Verification items for the finished model (mm, model axes). A direction names the side the tool comes from. Give positions to 0.01 mm unless a question says otherwise; leave off trailing zeros. Loops run counter-clockwise (first coordinate to the right, second up) from the corner with the lowest first, then second, coordinate; pieces in that order, holes last. Notation, with made-up numbers: M 20,-18 L 74,-18 A19 ccw 74,-11 Z; hole C 48.5,18 d9. An arc over 180 degrees is marked long. Use a Markdown table: item, result.
from build123d import *

# Parameters (mm, degrees)
SKETCH1_W           = 50
SKETCH1_H           = 101.6
BOSS_EXTRUDE1_DEPTH = 4
SKETCH2_R           = 3
CUT_EXTRUDE1_DEPTH  = 10
SKETCH3_R           = 6
CUT_EXTRUDE2_DEPTH  = 2


with BuildPart() as part:
    # Sketch1 → Boss-Extrude1 (new body)
    with BuildSketch(Plane(origin=(0, 0, 0), x_dir=(1, 0, 0), z_dir=(0, 1, 0))):
        Rectangle(SKETCH1_W, SKETCH1_H)
    extrude(amount=BOSS_EXTRUDE1_DEPTH)

    # Sketch2 → Cut-Extrude1 (cut)
    with BuildSketch(Plane(origin=(0, 4, 0), x_dir=(1, 0, 0), z_dir=(0, 1, 0))):
        with Locations((0, 20)):
            Circle(SKETCH2_R)
        with Locations((0, -20)):
            Circle(SKETCH2_R)
    extrude(amount=-CUT_EXTRUDE1_DEPTH, mode=Mode.SUBTRACT)

    # Sketch3 → Cut-Extrude2 (cut)
    with BuildSketch(Plane(origin=(0, 4, 0), x_dir=(1, 0, 0), z_dir=(0, 1, 0))):
        with Locations((0, 20)):
            Circle(SKETCH3_R)
        with Locations((0, -20)):
            Circle(SKETCH3_R)
    extrude(amount=-CUT_EXTRUDE2_DEPTH, mode=Mode.SUBTRACT)


solid = part.part
(1) Cross-section at C-C on y = 3. Record the cut outline in (x, z), then the cut area to 3 significant figures.
Results below:
| item | result |
|---|---|
| outline | M -25,-50.8 L 25,-50.8 L 25,50.8 L -25,50.8 Z; hole C 0,-20 d12; hole C 0,20 d12 |
| area | 4,850 mm^2 |
(2) Set-up check for faces 4 (the flat face through (0, 0, -1)), 5 (the cylindrical face through (-0.78, 3.01, 14.05)): record each of +Z, -Z, +X, -X, +Y, -Y from which the full face is reachable in a straight line by a thin tool's end or side.
Results below:
| item | result |
|---|---|
| face 4 | +Z, -Z, +X, -X, -Y |
| face 5 | +Y |
(3) Draft check along Z on faces 1 (the flat face through (0, 2, 50.8)), 2 (the flat face through (-25, 2, 1)), 3 (the cylindrical face through (-6, 3, -20)). Enter one of: +Z half, -Z half, draft (parallel to the pull), parting line (faces both ways), or undercut.
Results below:
| item | result |
|---|---|
| face 1 | +Z half |
| face 2 | draft |
| face 3 | undercut |
(4) Material ranges on line 1 (Z direction, x = 0, y = 0.8); line 2 (X direction, y = 2.85, z = 20); line 3 (X direction, y = 0.9, z = -20), recorded low to high.
Results below:
| item | result |
|---|---|
| line 1 | -50.8 to -23, -17 to 17, 23 to 50.8 |
| line 2 | -25 to -6, 6 to 25 |
| line 3 | -25 to -3, 3 to 25 |
(5) Cross-section at A-A on z = -20. Record the cut outline in (x, y), then the cut area to 3 significant figures.
Results below:
| item | result |
|---|---|
| outline | M -25,0 L -3,0 L -3,2 L -6,2 L -6,4 L -25,4 Z; M 3,0 L 25,0 L 25,4 L 6,4 L 6,2 L 3,2 Z |
| area | 164 mm^2 |
(6) Gauge pin test, flat end, axial feed: P1, Ø5, axis at x = 0, z = -20, coming from the +Y side. Record the tip position at first contact, or that the pin passes through.
Results below:
| item | result |
|---|---|
| P1 | through |
(7) Cross-section at B-B on x = 0. Record the cut outline in (y, z).
Results below:
| item | result |
|---|---|
| outline | M 0,-50.8 L 4,-50.8 L 4,-26 L 2,-26 L 2,-23 L 0,-23 Z; M 0,-17 L 2,-17 L 2,-14 L 4,-14 L 4,14 L 2,14 L 2,17 L 0,17 Z; M 0,23 L 2,23 L 2,26 L 4,26 L 4,50.8 L 0,50.8 Z |
